from build123d import *

# Parameters (mm, degrees)
F1_DEPTH = 12.7


with BuildPart() as f1:
    # F0 (on Top) → F1 (new body)
    with BuildSketch(Plane.XY):
        with BuildLine():
            ThreePointArc((0, 19.05), (13.470384, 13.470384), (19.05, 0))
            Line((19.05, 0), (19.05, -14.44625))
            ThreePointArc((19.05, -14.44625), (20.165923, -17.140327), (22.86, -18.25625))
            Line((22.86, -18.25625), (44.45, -18.25625))
            Line((44.45, -18.25625), (44.45, -14.675071))
            Line((44.45, -14.675071), (28.770535, -14.675071))
            add(Edge.make_bspline(
                [(22.225, 0), (22.447722, -8.768542), (22.86, -14.44625), (28.770535, -14.675071)],
                knots=[0, 0, 0, 0, 16.068657, 16.068657, 16.068657, 16.068657], degree=3))
            ThreePointArc((22.225, 0), (15.715448, 15.715448), (0, 22.225))
            ThreePointArc((0, 22.225), (-15.715448, 15.715448), (-22.225, 0))
            add(Edge.make_bspline(
                [(-22.225, 0), (-22.447722, -8.768542), (-22.86, -14.44625), (-28.770535, -14.675071)],
                knots=[0, 0, 0, 0, 16.068657, 16.068657, 16.068657, 16.068657], degree=3))
            Line((-28.770535, -14.675071), (-44.45, -14.675071))
            Line((-44.45, -14.675071), (-44.45, -18.25625))
            Line((-44.45, -18.25625), (-22.86, -18.25625))
            ThreePointArc((-22.86, -18.25625), (-20.165923, -17.140327), (-19.05, -14.44625))
            Line((-19.05, -14.44625), (-19.05, 0))
            ThreePointArc((-19.05, 0), (-13.470384, 13.470384), (0, 19.05))
        make_face()
    extrude(amount=F1_DEPTH)


solid = f1.part
Work out the finished part from the listing and answer in its coordinate system (mm). A direction names the side the tool comes from. Round coordinates to 2 decimals unless told otherwise and drop trailing zeros. Write each loop counter-clockwise with the first axis right and the second up, starting at its lowest first coordinate (ties: lowest second). Pieces come first, ordered by that corner, then holes. Notation, with made-up numbers: (-30.75, 54) -> (-16.75, 54) arc R29 ccw to (-16.75, 93) -> close; hole circle Ø10 at (16, 78.25). An arc over 180 degrees is marked (long way). Answer as CSV lines item,"result". Start each with the question number.
(1) Find the intervals of material crossed by probe 1 along Y at (x, z) = (34.5, 7.25); probe 2 along X at (y, z) = (9.5, 7.5); probe 3 along X at (y, z) = (-1, 10), in increasing order.
(2) Each of these flat-tipped pins is pushed along its axis until it touches: pin 1 (3 mm diameter, centred on y = 0.5, z = 3.5, fed in from +X); pin 2 (1.5 mm diameter, centred on x = 7.5, z = 7, fed in from +Y); pin 3 (4 mm diameter, centred on y = -5, z = 4, fed in from +X); pin 4 (6 mm diameter, centred on x = 7, y = 12.5, fed in from -Z). Where does it stop, or does it pass through?
(3) The part is cut by section A-A, the plane y = 10.5. Give the vertices of the cut face in (x, z), then the cut area to 3 significant figures.
(4) The part is cut by section C-C, the plane y = 6. Give the vertices of the cut face in (x, z).
(5) The mould has two halves that part along X. Classify faces 1 (the flat face through (-44.45, -16, 6)), 2 (the flat face through (19.05, -7, 6)), 3 (the flat face through (-34, -18.256, 6)), 4 (the cylindrical face through (20.136, -17.111, 6.261)): +X half, -X half, draft (parallel to the pull), parting line (faces both ways), or undercut.
(6) The part is cut by section B-B, the plane x = -34. Give the vertices of the cut face in (y, z), then the cut area to 3 significant figures.
(7) The part is cut by section D-D, the plane x = -4. Give the vertices of the cut face in (y, z), then the cut area to 3 significant figures.
(8) A tool of negligible diameter and unlimited length cuts with its end or side. For faces 5 (the cylindrical face through (-20.196, -17.17, 6.261)), 6 (the flat face through (-37, -14.675, 6)), 7 (the flat face through (37, -14.675, 6)), 8 (the flat face through (34, -18.256, 6)), from which of +Z, -Z, +X, -X, +Y, -Y can it reach the whole face along a straight path? Write none if from no direction.
Output values:
1,probe 1,"y = -18.26 to -14.68"
1,probe 2,"x = -20.09 to -16.51, 16.51 to 20.09"
1,probe 3,"x = -22.25 to -19.05, 19.05 to 22.25"
2,pin 1,"stops at x = 22.25"
2,pin 2,"stops at y = 21.18"
2,pin 3,"stops at x = 22.62"
2,pin 4,"passes through"
3,outline,"(-19.59, 0) -> (-15.9, 0) -> (-15.9, 12.7) -> (-19.59, 12.7) -> close; (15.9, 0) -> (19.59, 0) -> (19.59, 12.7) -> (15.9, 12.7) -> close"
3,area,"93.8 mm²"
4,outline,"(-21.4, 0) -> (-18.08, 0) -> (-18.08, 12.7) -> (-21.4, 12.7) -> close; (18.08, 0) -> (21.4, 0) -> (21.4, 12.7) -> (18.08, 12.7) -> close"
5,face 1,"-X half"
5,face 2,"undercut"
5,face 3,"draft"
5,face 4,"undercut"
6,outline,"(-18.26, 0) -> (-14.68, 0) -> (-14.68, 12.7) -> (-18.26, 12.7) -> close"
6,area,"45.5 mm²"
7,outline,"(18.63, 0) -> (21.86, 0) -> (21.86, 12.7) -> (18.63, 12.7) -> close"
7,area,"41.1 mm²"
8,face 5,"+Z, -Z, -Y"
8,face 6,"+Z, -Z, -X, +Y"
8,face 7,"+Z, -Z, +X, +Y"
8,face 8,"+Z, -Z, +X, -X, -Y"
